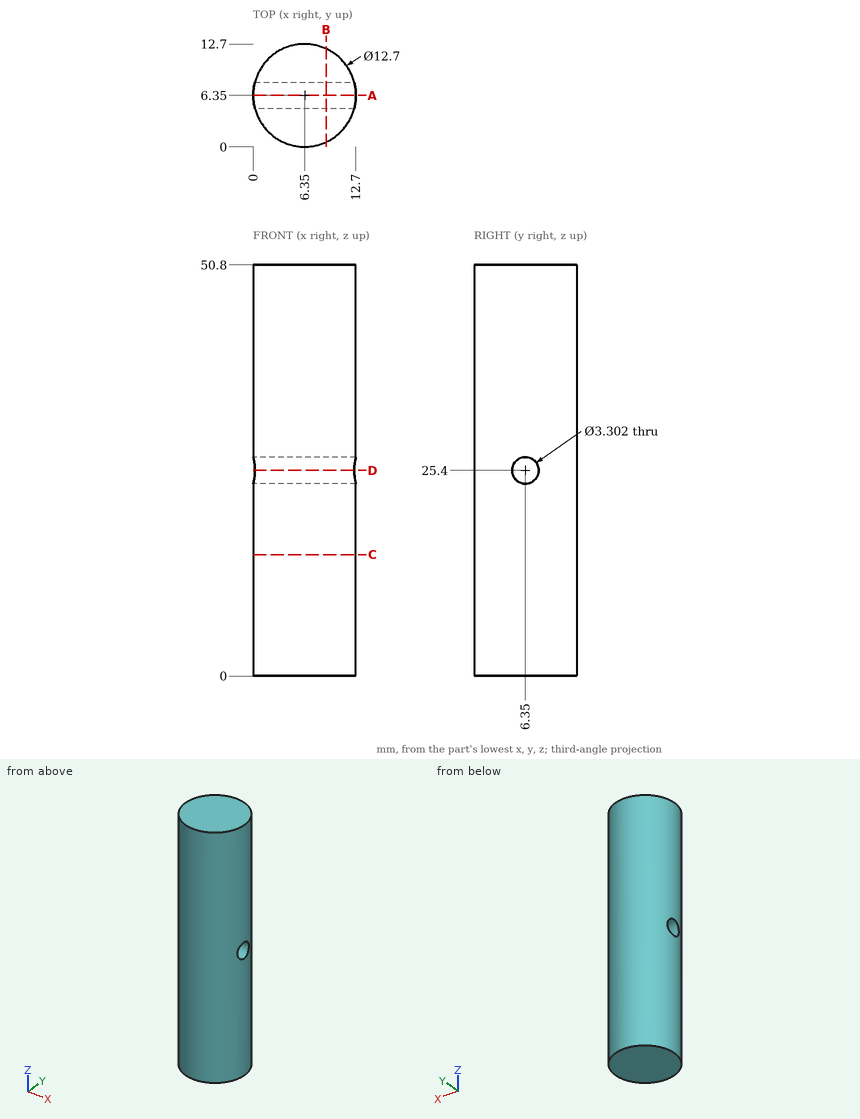
Job drawing, mm, ordinate dimensions from the low corner. One solid piece. Round coordinates to 2 decimals unless told otherwise and drop trailing zeros. Loops run counter-clockwise (first coordinate to the right, second up) from the corner with the lowest first, then second, coordinate; pieces in that order, holes last. Notation, with made-up numbers: (66, -3.5) -> (99, -3.5) arc R29 cw to (99, 31.5) -> close; hole circle Ø6 at (64, 84). An arc over 180 degrees is marked (long way). One line per item, written item: value. Start each with the question number.
Q1. Cut at D-D on z = 25.4. List the corners of the cut face in (x, y).
Q2. Cut at B-B on x = 9. List the corners of the cut face in (y, z), plus the area to 3 significant figures.
Q3. Cut at C-C on z = 15. List the corners of the cut face in (x, y).
Q4. Drop flat-ended pins along their axis: pin 1 Ø4 at (x, z) = (10.5, 39.5) entering from -Y; pin 2 Ø5 at (x, z) = (8.5, 5.5) entering from +Y; pin 3 Ø2 at (x, z) = (10, 21.5) entering from +Y; pin 4 Ø1.5 at (y, z) = (3.5, 10) entering from +X. Give the stop position or say it passes through.
Q5. Probe line 1 along Z through (x, y) = (3.25, 6.35); line 2 along Y through (x, z) = (11.5, 24); line 3 along Z through (x, y) = (8.5, 5.5). List the from-to ranges inside material, lowest first.
Q6. Cut at A-A on y = 6.35. List the corners of the cut face in (x, z), plus the area to 3 significant figures.
Computed:
1. outline: (0.22, 4.7) arc R6.35 ccw to (12.48, 4.7) -> close; (0.22, 8) -> (12.48, 8) arc R6.35 ccw to start
2. outline: (0.58, 0) -> (12.12, 0) -> (12.12, 50.8) -> (0.58, 50.8) -> close; hole circle Ø3.3 at (6.35, 25.4)
2. area: 578 mm²
3. outline: circle Ø12.7 at (6.35, 6.35)
4. pin 1: y = 0.38
4. pin 2: y = 12.7
4. pin 3: y = 12.12
4. pin 4: x = 12.34
5. line 1: 0 to 23.75, 27.05 to 50.8
5. line 2: 2.64 to 5.47, 7.23 to 10.06
5. line 3: 0 to 23.98, 26.82 to 50.8
6. outline: (0, 0) -> (12.7, 0) -> (12.7, 23.75) -> (0, 23.75) -> close; (0, 27.05) -> (12.7, 27.05) -> (12.7, 50.8) -> (0, 50.8) -> close
6. area: 603 mm²
